```python
from build123d import *

# Parameters (mm, degrees)
F0_W     = 100
F0_H     = 50
F1_DEPTH = 250
F2_R     = 25
F3_DEPTH = 15
F4_R     = 5
F5_T     = 2.5


with BuildPart() as f1:
    # F0 (on Top) → F1 (new body)
    with BuildSketch(Plane.XY):
        Rectangle(F0_W, F0_H)
    extrude(amount=F1_DEPTH)

    # F2 (on face) → F3 (join)
    with BuildSketch(Plane.XZ.offset(25)):
        with Locations((0, 210)):
            Circle(F2_R)
    extrude(amount=F3_DEPTH)

    # F4
    f4_edges = [f1.edges().sort_by_distance(p)[0] for p in [
        (-50, 0, 250),
        (0, 25, 250),
        (50, 0, 250),
        (0, -25, 250),
        (50, -25, 125),
        (50, 25, 125),
        (-50, -25, 125),
        (-50, 25, 125),
    ]]
    fillet(f4_edges, radius=F4_R)

    # F5
    f5_openings = [f1.faces().sort_by_distance(p)[0] for p in [
        (0, 0, 0),
    ]]
    offset(amount=F5_T, openings=f5_openings, kind=Kind.INTERSECTION)


solid = f1.part
```
CAD build for the part. Positions are in the model's coordinates, mm. A direction names the side the tool comes from. Round coordinates to 2 decimals unless told otherwise and drop trailing zeros. Order: outer loops, then holes, each group sorted by start corner. A loop starts at its lowest first (then second) coordinate and runs counter-clockwise, first axis right, second up. Notation, with made-up numbers: (43.5, 9) - (95.5, 9) arc R23 ccw to (95.5, 26) - close; hole circle Ø4 at (-5, -12). An arc over 180 degrees is marked (long way). Answer in a Markdown table with one row per item. Add a question column.
(1) 3-axis set-ups, long thin cutter, end or side, ignore diameter. For faces 4 (the face through (-1, 27.5, 121)), 5 (the face through (0, -40, 210)), 6 (the face through (-5.961, -34.895, 183.154)), 7 (the face through (-1, 0, 250)), 8 (the face through (0.63, -25.361, 250.245)): which of +Z, -Z, +X, -X, +Y, -Y reach the whole face in a straight line?
(2) Band-saw the part on B-B on z = 210. List the corners of the cut face in (x, y), and give its area (3 significant figures).
(3) Mould opens along X. For faces 1 (the face through (48, 24, 124)), 2 (the face through (50.245, -25.361, 124.215)), 3 (the face through (-52.5, 0, 121)) say: +X half, -X half, draft (parallel to the pull), parting line (faces both ways), or undercut.
(4) Drop flat-ended pins along their axis: pin 1 Ø5 at (x, z) = (-35.5, 54) entering from -Y; pin 2 Ø3 at (x, y) = (12.5, 16) entering from -Z; pin 3 Ø2 at (y, z) = (-25.5, 128) entering from -X. Give the stop position or say it passes through.
(5) Band-saw the part on A-A on x = -34. List the corners of the cut face in (y, z).
(6) Band-saw the part on D-D on z = 97.5. List the corners of the cut face in (x, y), and give its area (3 significant figures).
(7) Band-saw the part on C-C on y = 3.5. List the corners of the cut face in (x, z).
(8) Probe L1, parallel to Z at x = -1.5, y = -34; L2, parallel to X at y = -9, z = 176.5; L3, parallel to Y at x = 24.5, z = 82.5. List the from-to ranges inside material, lowest first. Write a range as [from, to].
Data:
| question | item | result |
|---|---|---|
| 1 | face 4 | +Z, -Z, +X, -X, +Y |
| 1 | face 5 | none |
| 1 | face 6 | -Y |
| 1 | face 7 | -Z |
| 1 | face 8 | +Z, +X, -X, -Y |
| 2 | outline | (-52.5, -20) arc R7.5 ccw to (-45, -27.5) - (-27.5, -27.5) - (-27.5, -42.5) - (27.5, -42.5) - (27.5, -27.5) - (45, -27.5) arc R7.5 ccw to (52.5, -20) - (52.5, 20) arc R7.5 ccw to (45, 27.5) - (-45, 27.5) arc R7.5 ccw to (-52.5, 20) - close; hole (-50, -20) arc R5 ccw to (-45, -25) - (-25, -25) - (-25, -40) - (25, -40) - (25, -25) - (45, -25) arc R5 ccw to (50, -20) - (50, 20) arc R5 ccw to (45, 25) - (-45, 25) arc R5 ccw to (-50, 20) - close |
| 2 | area | 823 mm^2 |
| 3 | face 1 | undercut |
| 3 | face 2 | +X half |
| 3 | face 3 | -X half |
| 4 | pin 1 | stops at y = -27.5 |
| 4 | pin 2 | stops at z = 250 |
| 4 | pin 3 | stops at x = -51 |
| 5 | outline | (-27.5, 0) - (-25, 0) - (-25, 245) arc R5 cw to (-20, 250) - (20, 250) arc R5 cw to (25, 245) - (25, 0) - (27.5, 0) - (27.5, 245) arc R7.5 ccw to (20, 252.5) - (-20, 252.5) arc R7.5 ccw to (-27.5, 245) - close |
| 6 | outline | (-52.5, -20) arc R7.5 ccw to (-45, -27.5) - (45, -27.5) arc R7.5 ccw to (52.5, -20) - (52.5, 20) arc R7.5 ccw to (45, 27.5) - (-45, 27.5) arc R7.5 ccw to (-52.5, 20) - close; hole (-50, -20) arc R5 ccw to (-45, -25) - (45, -25) arc R5 ccw to (50, -20) - (50, 20) arc R5 ccw to (45, 25) - (-45, 25) arc R5 ccw to (-50, 20) - close |
| 6 | area | 748 mm^2 |
| 7 | outline | (-52.5, 0) - (-50, 0) - (-50, 245) arc R5 cw to (-45, 250) - (45, 250) arc R5 cw to (50, 245) - (50, 0) - (52.5, 0) - (52.5, 245) arc R7.5 ccw to (45, 252.5) - (-45, 252.5) arc R7.5 ccw to (-52.5, 245) - close |
| 8 | L1 | z = [182.54, 185.05], [234.95, 237.46] |
| 8 | L2 | x = [-52.5, -50], [50, 52.5] |
| 8 | L3 | y = [-27.5, -25], [25, 27.5] |
